```python
from build123d import *

# Parameters (mm, degrees)
SM_BASE_FLANGE_1_DEPTH           = 1
OTHER_START                      = 68
OTHER_4_DEPTH                    = 35.5
OTHER_4_2_DEPTH                  = 35.5
CUT_EXTRUDE_1_REACH              = 134.863
SKETCH_10_R                      = 1.6
SM_EDGE_FLANGE_1_STRIP_W         = 5.4732
SM_EDGE_FLANGE_1_STRIP_H         = 1
SM_EDGE_FLANGE_1_STRIP_CUT_DEPTH = 154
SM_EDGE_FLANGE_1_DEPTH           = 154
SKETCH_14_W                      = 9.264116278
SKETCH_14_H                      = 12.510211191
CUT_EXTRUDE_2_DEPTH              = 133.863464967
CUT_EXTRUDE_3_REACH              = 190.904
SKETCH_15_W                      = 80
SKETCH_15_H                      = 29.662460086


# Read off the part's stored shape, not the designer's step: 绘制的折弯4
# Sheet-metal steps are written as plain solids
with BuildPart() as part:
    # Sketch 1 → 基体-法兰1 (new body)
    with BuildSketch(Plane(origin=(0, 0, 0), x_dir=(1, 0, 0), z_dir=(0, 1, 0))):
        Polygon((0.031889959, 65), (-77, 65), (-77, -65), (-32, -65), (-32, -68), (-55, -68), (-55, -103.5), (-14, -103.5), (-14, -106.5), (14, -106.5), (14, -103.5), (55, -103.5), (55, -68), (32, -68), (32, -65), (77, -65), (77, 65), align=None)
    extrude(amount=-SM_BASE_FLANGE_1_DEPTH)

    # Other 4 outline → Other 4 (cut)
    with BuildSketch(Plane.XY.offset(OTHER_START)):
        with BuildLine():
            Line((-55, -1), (-35.2634, -1))
            ThreePointArc((-35.2634, -1), (-36.195226164, -0.728828115), (-36.83604109, 0))
            Line((-36.83604109, 0), (-55, 0))
            Line((-55, 0), (-55, -1))
        make_face()
        with BuildLine():
            ThreePointArc((36.83604109, 0), (36.195226164, -0.728828115), (35.2634, -1))
            Line((35.2634, -1), (55, -1))
            Line((55, -1), (55, 0))
            Line((55, 0), (36.83604109, 0))
        make_face()
    extrude(amount=OTHER_4_DEPTH, mode=Mode.SUBTRACT)

    # Other 4 2 outline → Other 4 2 (add)
    with BuildSketch(Plane.XY.offset(OTHER_START)):
        with BuildLine():
            ThreePointArc((-37, 0.7366), (-36.958514757, 0.359286442), (-36.83604109, 0))
            Line((-36.83604109, 0), (-35.2634, 0))
            ThreePointArc((-35.2634, 0), (-35.784254855, 0.215745145), (-36, 0.7366))
            Line((-36, 0.7366), (-36, 18.530753262))
            Line((-36, 18.530753262), (-37, 18.530753262))
            Line((-37, 18.530753262), (-37, 0.7366))
        make_face()
        with BuildLine():
            Line((35.2634, 0), (36.83604109, 0))
            ThreePointArc((36.83604109, 0), (36.958514757, 0.359286442), (37, 0.7366))
            Line((37, 0.7366), (37, 18.530753262))
            Line((37, 18.530753262), (36, 18.530753262))
            Line((36, 18.530753262), (36, 0.7366))
            ThreePointArc((36, 0.7366), (35.784254855, 0.215745145), (35.2634, 0))
        make_face()
    extrude(amount=OTHER_4_2_DEPTH)

    # 草图10 → 切除-拉伸1 (cut, up to next)
    with BuildSketch(Plane.XZ.offset(1), mode=Mode.PRIVATE) as cut_extrude_1_sk1:
        with Locations(Location((-72, -51.5, 0), (0, 0, 270))):
            Circle(SKETCH_10_R)
    cut_extrude_1_tool1 = extrude(cut_extrude_1_sk1.sketch, amount=-CUT_EXTRUDE_1_REACH, mode=Mode.PRIVATE) & part.part
    # 草图10 → 切除-拉伸1 (cut, up to next)
    with BuildSketch(Plane.XZ.offset(1), mode=Mode.PRIVATE) as cut_extrude_1_sk2:
        with Locations(Location((-72, 51.5, 0), (0, 0, 270))):
            Circle(SKETCH_10_R)
    cut_extrude_1_tool2 = extrude(cut_extrude_1_sk2.sketch, amount=-CUT_EXTRUDE_1_REACH, mode=Mode.PRIVATE) & part.part
    # 草图10 → 切除-拉伸1 (cut, up to next)
    with BuildSketch(Plane.XZ.offset(1), mode=Mode.PRIVATE) as cut_extrude_1_sk3:
        with Locations(Location((72, -51.5, 0), (0, 0, 270))):
            Circle(SKETCH_10_R)
    cut_extrude_1_tool3 = extrude(cut_extrude_1_sk3.sketch, amount=-CUT_EXTRUDE_1_REACH, mode=Mode.PRIVATE) & part.part
    # 草图10 → 切除-拉伸1 (cut, up to next)
    with BuildSketch(Plane.XZ.offset(1), mode=Mode.PRIVATE) as cut_extrude_1_sk4:
        with Locations(Location((72, 51.5, 0), (0, 0, 270))):
            Circle(SKETCH_10_R)
    cut_extrude_1_tool4 = extrude(cut_extrude_1_sk4.sketch, amount=-CUT_EXTRUDE_1_REACH, mode=Mode.PRIVATE) & part.part
    add(cut_extrude_1_tool1.solids().sort_by_distance((-72, -1, -51.5))[0], mode=Mode.SUBTRACT)
    add(cut_extrude_1_tool2.solids().sort_by_distance((-72, -1, 51.5))[0], mode=Mode.SUBTRACT)
    add(cut_extrude_1_tool3.solids().sort_by_distance((72, -1, -51.5))[0], mode=Mode.SUBTRACT)
    add(cut_extrude_1_tool4.solids().sort_by_distance((72, -1, 51.5))[0], mode=Mode.SUBTRACT)

    # 边线-法兰1 strip (across the edge) → 边线-法兰1 strip cut (cut)
    with BuildSketch(Plane(origin=(77, 0, -65), x_dir=(0, 0, 1), z_dir=(-1, 0, 0))):
        with Locations((-1, -0.5)):
            Rectangle(SM_EDGE_FLANGE_1_STRIP_W, SM_EDGE_FLANGE_1_STRIP_H)
    extrude(amount=SM_EDGE_FLANGE_1_STRIP_CUT_DEPTH, mode=Mode.SUBTRACT)

    # 边线-法兰1 section (across the edge) → 边线-法兰1 (add)
    with BuildSketch(Plane(origin=(77, 0, -65), x_dir=(0, 0, 1), z_dir=(-1, 0, 0))):
        with BuildLine():
            Line((0, 0.7366), (0, 17))
            Line((0, 17), (1, 17))
            Line((1, 17), (1, 0.7366))
            ThreePointArc((1, 0.7366), (1.215745145, 0.215745145), (1.7366, 0))
            Line((1.7366, 0), (1.7366, -1))
            ThreePointArc((1.7366, -1), (0.508638364, -0.491361636), (0, 0.7366))
        make_face()
    extrude(amount=SM_EDGE_FLANGE_1_DEPTH)

    # 草图14 → 切除-拉伸2 (cut, through all)
    with BuildSketch(Plane.XZ.offset(1)):
        with Locations((-78.632058139, -66.255105596)):
            Rectangle(SKETCH_14_W, SKETCH_14_H)
        with Locations((78.632058139, -66.255105596)):
            Rectangle(SKETCH_14_W, SKETCH_14_H)
    extrude(amount=-CUT_EXTRUDE_2_DEPTH, mode=Mode.SUBTRACT)

    # 草图15 → 切除-拉伸3 (cut, up to next)
    with BuildSketch(Plane(origin=(0, 0, -65), x_dir=(-1, 0, 0), z_dir=(0, 0, -1)), mode=Mode.PRIVATE) as cut_extrude_3_sk1:
        with Locations((0, 26.831230043)):
            Rectangle(SKETCH_15_W, SKETCH_15_H)
    cut_extrude_3_tool1 = extrude(cut_extrude_3_sk1.sketch, amount=-CUT_EXTRUDE_3_REACH, mode=Mode.PRIVATE) & part.part
    add(cut_extrude_3_tool1.solids().sort_by_distance((0, 26.83123, -65))[0], mode=Mode.SUBTRACT)


solid = part.part
```
Model file for the job. Use its own axes, mm. A direction names the side the tool comes from. Coordinates: 2 decimals unless noted, no trailing zeros. Write each loop counter-clockwise with the first axis right and the second up, starting at its lowest first coordinate (ties: lowest second). Pieces come first, ordered by that corner, then holes. Notation, with made-up numbers: (80, 85) - (99, 85) arc R13 cw to (99, 110) - close; hole circle Ø9 at (-20.5, 84). An arc over 180 degrees is marked (long way). One line per question, with ' | ' between items. Start each with the question number.
Q1. Cut at D-D, the plane x = 45.5. List the corners of the cut face in (y, z).
Q2. Pull direction Z, two halves, no side cores. Call faces 5 (the face through (30.6, -0.6, 103.5)), 6 (the face through (-36.2, 7.4, 68)), 7 (the face through (1, 7, -65)): pulls with the +Z half, pulls with the -Z half, needs draft (parallel to the pull), parting line crosses it, or undercut.
Q3. Pin check, flat tips, straight feed: pin 1 (2 mm diameter, centred on x = 28.5, y = 1.5, fed in from +Z); pin 2 (0.8 mm diameter, centred on x = -17, z = -64.5, fed in from +Y); pin 3 (3.5 mm diameter, centred on x = 72, z = 51.5, fed in from +Y). Stop position of each tip, or through.
Q4. Cut at C-C, the plane z = 78.5. List the corners of the cut face in (x, y).
Q5. Drill centre lines: line 1 (X direction, y = -0.65, z = -51.5); line 2 (Z direction, x = -72, y = -0.7); line 3 (Z direction, x = 72, y = -0.5). Where is each one in solid material? Low to high. Write a range as [from, to].
Q6. 3-axis set-ups, long thin cutter, end or side, ignore diameter. For faces 1 (the face through (-74, 6, -64.2)), 2 (the face through (36.2, 7.4, 68)), 3 (the face through (-37, 10, 86)), 4 (the face through (36, 10, 86)): which of +Z, -Z, +X, -X, +Y, -Y reach the whole face in a straight line?
Q7. Cut at A-A, the plane y = 3.75. List the corners of the cut face in (x, z), then the cut area to 3 significant figures.
Q8. Cut at B-B, the plane x = -18. List the corners of the cut face in (y, z), then the cut area to 3 significant figures.
Answer below:
1) outline: (-1, -63.26) arc R1.74 ccw to (0.74, -65) - (17, -65) - (17, -64) - (0.74, -64) arc R0.74 cw to (0, -63.26) - (0, 65) - (-1, 65) - close
2) face 5: pulls with the +Z half | face 6: undercut | face 7: pulls with the -Z half
3) pin 1: z = -63.96 | pin 2: y = 12 | pin 3: y = 0
4) outline: (-37, 0.74) arc R1.74 ccw to (-35.26, -1) - (35.26, -1) arc R1.74 ccw to (37, 0.74) - (37, 18.53) - (36, 18.53) - (36, 0.74) arc R0.74 cw to (35.26, 0) - (-35.26, 0) arc R0.74 cw to (-36, 0.74) - (-36, 18.53) - (-37, 18.53) - close
5) line 1: [-77, -73.6], [-70.4, 70.4], [73.6, 77] | line 2: [-64.24, -53.1], [-49.9, 49.9], [53.1, 65] | line 3: [-64.48, -53.1], [-49.9, 49.9], [53.1, 65]
6) face 1: -Z, -X, +Y, -Y | face 2: +X, +Y, -Y | face 3: +Z, -X, +Y, -Y | face 4: +Z, +Y
7) outline: (-74, -65) - (74, -65) - (74, -64) - (-74, -64) - close; (-37, 68) - (-36, 68) - (-36, 103.5) - (-37, 103.5) - close; (36, 68) - (37, 68) - (37, 103.5) - (36, 103.5) - close | area: 219 mm^2
8) outline: (-1, -63.26) arc R1.74 ccw to (0.74, -65) - (12, -65) - (12, -64) - (0.74, -64) arc R0.74 cw to (0, -63.26) - (0, 103.5) - (-1, 103.5) - close | area: 180 mm^2
